Design review of the part built by this model. Coordinates are the model's own, in mm. A direction names the side the tool comes from. Give positions to 0.01 mm unless a question says otherwise; leave off trailing zeros. Write each loop counter-clockwise with the first axis right and the second up, starting at its lowest first coordinate (ties: lowest second). Pieces come first, ordered by that corner, then holes. Notation, with made-up numbers: (-16, -2) - (36, -2) arc R9 ccw to (36, 6) - close; hole circle Ø2 at (45.5, -13). An arc over 180 degrees is marked (long way). Write each question's results on one line, items separated by ' | '. Start each with the question number.
from build123d import *

# Parameters (mm, degrees)
F0_R     = 40
F1_DEPTH = 80
F3_DEPTH = 7.5


with BuildPart() as f1:
    # F0 (on Top) → F1 (new body)
    with BuildSketch(Plane.XY):
        Circle(F0_R)
    extrude(amount=F1_DEPTH)

    # F2 (on Front) → F3 (cut, symmetric)
    with BuildSketch(Plane.XZ):
        with BuildLine():
            Line((-40, 80), (-40, 0))
            Line((-40, 0), (6.54234, 0))
            Line((6.54234, 0), (6.54234, 18.178894))
            Line((6.54234, 18.178894), (-8.40058, 16.871557))
            ThreePointArc((-8.40058, 16.871557), (-17.49097, 6.038053), (-28.324474, 15.128443))
            Line((-28.324474, 15.128443), (-34, 80))
            Line((-34, 80), (-40, 80))
        make_face()
    extrude(amount=F3_DEPTH, both=True, mode=Mode.SUBTRACT)


solid = f1.part
Q1. The part is to be moulded in two halves that separate along Y. For faces 1 (the face through (6.542, 0, 9)), 2 (the face through (39.966, -1.653, 39.44)), 3 (the face through (-31.123, -0.105, 47.11)), 4 (the face through (0, 1, 80)), say which applies: +Y half, -Y half, draft (parallel to the pull), parting line (faces both ways), or undercut.
Q2. Add section D-D on x = -19.5. State the section outline as (y, z) points.
Q3. For line 1 along Y through (x, z) = (-1, 65); line 2 along Y through (x, z) = (-34, 26); line 3 along X through (y, z) = (-24.5, 4), list the stretches that pass through material, from the lowest coordinate up. Write a range as [from, to].
Q4. Add section B-B on y = 1.5. State the section outline as (x, z) points.
Q5. Insertion check: P1, Ø1, axis at x = -26.5, z = 59.5, coming from the +Y side; P2, Ø1.5, axis at y = 8.5, z = 57.5, coming from the +X side; P3, Ø8, axis at x = -23.5, y = -26, coming from the -Z side; P4, Ø2, axis at y = -31.5, z = 17, coming from the -X side. Each pin has a flat end and moves straight along its axis. Give the tip position at first contact, or say it passes through.
Q6. Add section A-A on z = 12.5. State the section outline as (x, y) points.
Q7. Machinability: for faces 5 (the face through (9, 1, 0)), 6 (the face through (-30, -7.5, 22)), which of the approach directions +Z, -Z, +X, -X, +Y, -Y give a long, thin tool a straight path to every point of the face, cutting with its end or side? Answer none if there is none.
Q8. Add section C-C on x = -32. State the section outline as (y, z) points, plus the area to 3 significant figures.
Result:
1) face 1: undercut | face 2: parting line | face 3: undercut | face 4: draft
2) outline: (-34.92, 0) - (-7.5, 0) - (-7.5, 6.06) - (7.5, 6.06) - (7.5, 0) - (34.92, 0) - (34.92, 80) - (-34.92, 80) - close
3) line 1: y = [-39.99, 39.99] | line 2: y = [-21.07, -7.5], [7.5, 21.07] | line 3: x = [-31.62, 31.62]
4) outline: (-34, 80) - (-28.32, 15.13) arc R10 ccw to (-8.4, 16.87) - (6.54, 18.18) - (6.54, 0) - (39.97, 0) - (39.97, 80) - close
5) P1: stops at y = 30.4 | P2: stops at x = 39.24 | P3: stops at z = 0 | P4: stops at x = -25.88
6) outline: (-39.29, -7.5) arc R40 ccw (long way) to (-39.29, 7.5) - (-27.73, 7.5) - (-27.73, -7.5) - close; hole (-9, -7.5) - (6.54, -7.5) - (6.54, 7.5) - (-9, 7.5) - close
7) face 5: -Z, +X, -X, +Y, -Y | face 6: -Z
8) outline: (-24, 0) - (-7.5, 0) - (-7.5, 57.14) - (7.5, 57.14) - (7.5, 0) - (24, 0) - (24, 80) - (-24, 80) - close | area: 2,980 mm²
